from build123d import *

# Parameters (mm, degrees)
SKETCH1_W           = 51.15
SKETCH1_H           = 28
BOSS_EXTRUDE1_DEPTH = 1.6
SKETCH2_R           = 1
CUT_EXTRUDE1_DEPTH  = 30.200010702
FILLET1_R           = 2
SKETCH3_W           = 18.25
SKETCH3_H           = 9
BOSS_EXTRUDE2_DEPTH = 2.36


with BuildPart() as part:
    # Sketch1 → Boss-Extrude1 (new body)
    with BuildSketch(Plane(origin=(0, 0, 0), x_dir=(1, 0, 0), z_dir=(0, 1, 0))):
        Rectangle(SKETCH1_W, SKETCH1_H)
    extrude(amount=BOSS_EXTRUDE1_DEPTH)

    # Sketch2 → Cut-Extrude1 (cut, through all)
    with BuildSketch(Plane(origin=(0, 1.6, 0), x_dir=(1, 0, 0), z_dir=(0, 1, 0))):
        with Locations(Location((-24.075, 12.5, 0), (0, 0, 270))):
            Circle(SKETCH2_R)
        with Locations(Location((24.075, 12.5, 0), (0, 0, 270))):
            Circle(SKETCH2_R)
        with Locations(Location((24.075, -12.5, 0), (0, 0, 270))):
            Circle(SKETCH2_R)
        with Locations(Location((-24.075, -12.5, 0), (0, 0, 270))):
            Circle(SKETCH2_R)
    extrude(amount=-CUT_EXTRUDE1_DEPTH, mode=Mode.SUBTRACT)

    # Fillet1
    fillet1_edges = [part.edges().sort_by_distance(p)[0] for p in [
        (-25.575, 0.8, -14),
        (25.575, 0.8, -14),
        (25.575, 0.8, 14),
        (-25.575, 0.8, 14),
    ]]
    fillet(fillet1_edges, radius=FILLET1_R)

    # Sketch3 → Boss-Extrude2 (add)
    with BuildSketch(Plane.XZ):
        Rectangle(SKETCH3_W, SKETCH3_H)
    extrude(amount=BOSS_EXTRUDE2_DEPTH)


solid = part.part
The listing builds one solid part. Answer for the finished solid, in the listing's coordinates (mm). A direction names the side the tool comes from. Round coordinates to 2 decimals unless told otherwise and drop trailing zeros. Write each loop counter-clockwise with the first axis right and the second up, starting at its lowest first coordinate (ties: lowest second). Pieces come first, ordered by that corner, then holes. Notation, with made-up numbers: M -31.5,76 L -18.5,76 A22 cw -18.5,115 Z; hole C 28.5,76 d8. An arc over 180 degrees is marked long. Write each question's results on one line, items separated by ' | '. Start each with the question number.
(1) Find the intervals of material crossed by line 1 (X direction, y = 1.15, z = -12.5) (1 decimal); line 2 (Y direction, x = -12.5, z = 13.25); line 3 (Z direction, x = -7, y = -1.9), in increasing order.
(2) The part is cut by section A-A, the plane x = 3.5. Write down the section's boundary in (y, z), and give its area (3 significant figures).
(3) Determine the mould class of faces 5 (the flat face through (-25.575, 1, 0)), 6 (the cylindrical face through (23.188, 0.811, -12.039)), 7 (the flat face through (0, 1, -14)) for opening direction X: +X half, -X half, draft (parallel to the pull), parting line (faces both ways), or undercut.
(4) The part is cut by section D-D, the plane y = -1. Write down the section's boundary in (x, z) (3 decimals), and give its area (3 significant figures).
(5) The part is cut by section B-B, the plane z = 2. Write down the section's boundary in (x, y) (3 decimals).
(6) For faces 1 (the flat face through (-9.125, -1, 0)), 2 (the flat face through (0, -1, 4.5)), 3 (the flat face through (0, -1, -4.5)), 4 (the flat face through (9.125, -1, 0)), determine the directions among +Z, -Z, +X, -X, +Y, -Y from which every point of the face is accessible in a straight line to the end or side of a thin tool.
(7) Each of these flat-tipped pins is pushed along its axis until it touches: P1, Ø1.9, axis at y = -1, z = -0.5, coming from the -X side (3 decimals); P2, Ø2.5, axis at x = -24.075, z = -12.5, coming from the -Y side; P3, Ø1.8, axis at x = 24.075, z = -12.5, coming from the +Y side; P4, Ø2, axis at x = 4, y = -1.5, coming from the +Z side. Where does it stop, or does it pass through?
(8) The part is cut by section C-C, the plane z = -12.5. Write down the section's boundary in (x, y) (1 decimal).
Worked answers:
1) line 1: x = -25.5 to -25.1, -23.1 to 23.1, 25.1 to 25.5 | line 2: y = 0 to 1.6 | line 3: z = -4.5 to 4.5
2) outline: M -2.36,-4.5 L 0,-4.5 L 0,-14 L 1.6,-14 L 1.6,14 L 0,14 L 0,4.5 L -2.36,4.5 Z | area: 66.0 mm²
3) face 5: -X half | face 6: undercut | face 7: draft
4) outline: M -9.125,-4.5 L 9.125,-4.5 L 9.125,4.5 L -9.125,4.5 Z | area: 164 mm²
5) outline: M -25.575,0 L -9.125,0 L -9.125,-2.36 L 9.125,-2.36 L 9.125,0 L 25.575,0 L 25.575,1.6 L -25.575,1.6 Z
6) face 1: +Z, -Z, -X, -Y | face 2: +Z, +X, -X, -Y | face 3: -Z, +X, -X, -Y | face 4: +Z, -Z, +X, -Y
7) P1: stops at x = -9.125 | P2: stops at y = 0 | P3: passes through | P4: stops at z = 4.5
8) outline: M -25.5,0 L -25.1,0 L -25.1,1.6 L -25.5,1.6 Z; M -23.1,0 L 23.1,0 L 23.1,1.6 L -23.1,1.6 Z; M 25.1,0 L 25.5,0 L 25.5,1.6 L 25.1,1.6 Z
